from build123d import *

# Parameters (mm, degrees)
SZKIC1_R                               = 47.5
DODANIE_WYCI_GNI_CIE1_DEPTH            = 30
WYTNIJ_WYCI_GNI_CIE1_REACH             = 75.57
SZKIC2_R                               = 5
SZYK_KO_OWY1_COUNT                     = 6
SZKIC3_R                               = 21
DODANIE_WYCI_GNI_CIE2_DEPTH            = 585
DODANIE_WYCI_GNI_CIE3_DEPTH            = 75
SZKIC5_R                               = 22
DODANIE_WYCI_GNI_CIE4_DEPTH            = 3
SZKIC7_R                               = 21
DODANIE_WYCI_GNI_CIE5_DEPTH            = 5
WYTNIJ_WYCI_GNI_CIE2_REACH             = 696.362
SZKIC8_R                               = 10
WYTNIJ_WYCI_GNI_CIE2_DIRECTION_2_DEPTH = 695.361937321
WYTNIJ_WYCI_GNI_CIE3_START             = -67
WYTNIJ_WYCI_GNI_CIE3_DEPTH             = 67
ZAOKR_GLENIE1_R                        = 8


with BuildPart() as part:
    # Szkic1 → Dodanie-wyciągnięcie1 (new body)
    with BuildSketch(Plane.XY):
        Circle(SZKIC1_R)
    extrude(amount=DODANIE_WYCI_GNI_CIE1_DEPTH)

    # Szkic2 → Wytnij-wyciągnięcie1 (cut, up to next)
    with BuildSketch(Plane.XY.offset(30), mode=Mode.PRIVATE) as wytnij_wyci_gni_cie1_sk1:
        with Locations((0, 41.25)):
            Circle(SZKIC2_R)
    wytnij_wyci_gni_cie1_tool1 = extrude(wytnij_wyci_gni_cie1_sk1.sketch, amount=-WYTNIJ_WYCI_GNI_CIE1_REACH, mode=Mode.PRIVATE) & part.part
    wytnij_wyci_gni_cie1 = wytnij_wyci_gni_cie1_tool1.solids().sort_by_distance((0, 41.25, 30))[0]
    add(wytnij_wyci_gni_cie1, mode=Mode.SUBTRACT)

    # Szyk kołowy1: Wytnij-wyciągnięcie1 ×6 about axis
    szyk_ko_owy1_axis = Axis((0, 0, 0), (0, 0, 1))
    for i in range(1, SZYK_KO_OWY1_COUNT):
        add(wytnij_wyci_gni_cie1.rotate(szyk_ko_owy1_axis, i * 360 / SZYK_KO_OWY1_COUNT), mode=Mode.SUBTRACT)

    # Szkic3 → Dodanie-wyciągnięcie2 (add)
    with BuildSketch(Plane.XY.offset(30)):
        Circle(SZKIC3_R)
    extrude(amount=DODANIE_WYCI_GNI_CIE2_DEPTH)

    # Szkic4 → Dodanie-wyciągnięcie3 (add)
    with BuildSketch(Plane.XY.offset(615)):
        with BuildLine():
            Line((-15.652475842, 14), (15.652475842, 14))
            ThreePointArc((15.652475842, 14), (0, 21), (-15.652475842, 14))
        make_face()
        with BuildLine():
            Line((-15.652475842, -14), (15.652475842, -14))
            ThreePointArc((15.652475842, -14), (0, -21), (-15.652475842, -14))
        make_face()
    extrude(amount=DODANIE_WYCI_GNI_CIE3_DEPTH)

    # Szkic5 → Dodanie-wyciągnięcie4 (add)
    with BuildSketch(Plane.XY.offset(615)):
        Circle(SZKIC5_R)
    extrude(amount=DODANIE_WYCI_GNI_CIE4_DEPTH)

    # Szkic7 → Dodanie-wyciągnięcie5 (add)
    with BuildSketch(Plane.XY.offset(618)):
        Circle(SZKIC7_R)
    extrude(amount=DODANIE_WYCI_GNI_CIE5_DEPTH)

    # Szkic8 → Wytnij-wyciągnięcie2 (cut, up to next)
    with BuildSketch(Plane(origin=(0, -14, 0), x_dir=(1, 0, 0), z_dir=(0, 1, 0)), mode=Mode.PRIVATE) as wytnij_wyci_gni_cie2_sk1:
        with Locations(Location((0, -675, 0), (0, 0, 90))):
            Circle(SZKIC8_R)
    wytnij_wyci_gni_cie2_tool1 = extrude(wytnij_wyci_gni_cie2_sk1.sketch, amount=-WYTNIJ_WYCI_GNI_CIE2_REACH, mode=Mode.PRIVATE) & part.part
    add(wytnij_wyci_gni_cie2_tool1.solids().sort_by_distance((0, -14, 675))[0], mode=Mode.SUBTRACT)

    # Szkic8 → Wytnij-wyciągnięcie2 direction 2 (cut)
    with BuildSketch(Plane(origin=(0, -14, 0), x_dir=(1, 0, 0), z_dir=(0, 1, 0))):
        with Locations(Location((0, -675, 0), (0, 0, 90))):
            Circle(SZKIC8_R)
    extrude(amount=WYTNIJ_WYCI_GNI_CIE2_DIRECTION_2_DEPTH, mode=Mode.SUBTRACT)

    # Szkic9 → Wytnij-wyciągnięcie3 (cut)
    with BuildSketch(Plane.XY.offset(690).offset(WYTNIJ_WYCI_GNI_CIE3_START)):
        with BuildLine():
            Line((-11.652475842, 14), (-11.652475842, 17.470541112))
            ThreePointArc((-11.652475842, 17.470541112), (-13.762313052, 15.861864312), (-15.652475842, 14))
            Line((-15.652475842, 14), (-11.652475842, 14))
        make_face()
        with BuildLine():
            Line((15.652475842, 14), (11.652475842, 14))
            Line((11.652475842, 14), (11.652475842, 17.470541112))
            ThreePointArc((11.652475842, 17.470541112), (13.762313052, 15.861864312), (15.652475842, 14))
        make_face()
        with BuildLine():
            Line((11.652475842, -14), (11.652475842, -17.470541112))
            ThreePointArc((11.652475842, -17.470541112), (13.762313052, -15.861864312), (15.652475842, -14))
            Line((15.652475842, -14), (11.652475842, -14))
        make_face()
        with BuildLine():
            Line((-15.652475842, -14), (-11.652475842, -14))
            Line((-11.652475842, -14), (-11.652475842, -17.470541112))
            ThreePointArc((-11.652475842, -17.470541112), (-13.762313052, -15.861864312), (-15.652475842, -14))
        make_face()
    extrude(amount=WYTNIJ_WYCI_GNI_CIE3_DEPTH, mode=Mode.SUBTRACT)

    # Zaokrąglenie1
    # the kernel refuses this fillet: 8 mm, written as the material it adds along each edge
    with BuildSketch(Plane(origin=(-11.652475842, -14, 623), x_dir=(0, 1, 0), z_dir=(1, 0, 0))) as zaokr_glenie1_piece_1:
        with BuildLine():
            CenterArc((ZAOKR_GLENIE1_R, ZAOKR_GLENIE1_R), ZAOKR_GLENIE1_R, 180, 90)
            Line((0, ZAOKR_GLENIE1_R), (0, 0))
            Line((0, 0), (ZAOKR_GLENIE1_R, 0))
        make_face()
    extrude(amount=23.304951685)
    with BuildSketch(Plane(origin=(-11.652475842, 14, 623), x_dir=(0, -1, 0), z_dir=(1, 0, 0))) as zaokr_glenie1_piece_2:
        with BuildLine():
            CenterArc((ZAOKR_GLENIE1_R, -ZAOKR_GLENIE1_R), ZAOKR_GLENIE1_R, 90, 90)
            Line((0, -ZAOKR_GLENIE1_R), (0, 0))
            Line((0, 0), (ZAOKR_GLENIE1_R, 0))
        make_face()
    extrude(amount=23.304951685)


solid = part.part
Design review of the part built by this model. Coordinates are the model's own, in mm. A direction names the side the tool comes from. Round coordinates to 2 decimals unless told otherwise and drop trailing zeros. Write each loop counter-clockwise with the first axis right and the second up, starting at its lowest first coordinate (ties: lowest second). Pieces come first, ordered by that corner, then holes.
Item 1: Consider section A-A on z = 675. Give the boundary of the cut face in (x, y).
Item 2: For faces 1 (the cylindrical face through (-4.769, -21.477, 616.479)), 2 (the flat face through (-11.652, 16, 654)), 3 (the cylindrical face through (20.03, 6.31, 318.4)), 4 (the flat face through (0, 14, 654)), 5 (the flat face through (11.652, 16, 654)), list the 3-axis set-ups (+Z, -Z, +X, -X, +Y, -Y) from which the entire face can be reached by the end or side of a thin tool; tool diameter is ignored.
Item 3: For pin 1 Ø2 at (y, z) = (9, 78) entering from -X; pin 2 Ø8 at (x, y) = (-35.72, -20.62) entering from +Z; pin 3 Ø4 at (y, z) = (13, 179.5) entering from -X; pin 4 Ø12.5 at (y, z) = (9.5, 648.5) entering from -X, all flat-tipped, find the tip position at first contact; note any pin that passes through.
Item 4: Draft analysis for pull direction Z (two halves, no side actions). For faces 6 (the flat face through (11.652, -16, 654)), 7 (the flat face through (-1, 1, 0)), 8 (the cylindrical face through (-3, 16.67, 665.46)), state which applies: released by +Z, released by -Z, zero draft, split by the parting line, or undercut.
Item 5: Wall thickness on L1, parallel to X at y = 17, z = 675; L2, parallel to Z at x = 12, y = 31.5; L3, parallel to Y at x = -18.5, z = 53: over which ranges is each line inside the solid? List them lowest first.
Item 6: Consider section B-B on z = 367. Give the boundary of the cut face in (x, y), and give its area (3 significant figures).
Check values:
1. outline: (-11.65, -17.47) arc R21 ccw to (-10, -18.47) - (-10, -14) - (-11.65, -14) - close; (-11.65, 14) - (-10, 14) - (-10, 18.47) arc R21 ccw to (-11.65, 17.47) - close; (10, -18.47) arc R21 ccw to (11.65, -17.47) - (11.65, -14) - (10, -14) - close; (10, 14) - (11.65, 14) - (11.65, 17.47) arc R21 ccw to (10, 18.47) - close
2. face 1: +Z
2. face 2: +Z, -X, +Y, -Y
2. face 3: none
2. face 4: +Z, +X, -X
2. face 5: +Z, +X, +Y, -Y
3. pin 1: stops at x = -19.42
3. pin 2: passes through
3. pin 3: stops at x = -17.89
3. pin 4: stops at x = -11.65
4. face 6: zero draft
4. face 7: released by -Z
4. face 8: undercut
5. L1: x = -11.65 to -10, 10 to 11.65
5. L2: z = 0 to 30
5. L3: y = -9.94 to 9.94
6. outline: circle Ø42 at (0, 0)
6. area: 1,390 mm2
